Read the model definition and answer for the solid it produces. Units are mm, in the model's axes. A direction names the side the tool comes from. Coordinates: 2 decimals unless noted, no trailing zeros. Write each loop counter-clockwise with the first axis right and the second up, starting at its lowest first coordinate (ties: lowest second). Pieces come first, ordered by that corner, then holes.
Item 1: Section B-B (y = 7) is taken. Give the vertices of the cut face in (x, z), then the cut area to 3 significant figures.
Item 2: Each of these flat-tipped pins is pushed along its axis until it touches: P1, Ø3, axis at x = -1, y = 33, coming from the -Z side; P2, Ø1, axis at x = -4.5, y = 35, coming from the +Z side. Where does it stop, or does it pass through?
Item 3: A tool of negligible diameter and unlimited length cuts with its end or side. For faces 1 (the face through (7, 1, -43)), 2 (the face through (-6, 29, 40)), 3 (the face through (3.5, 2, 41)), 4 (the face through (3.5, 2, -41)), 5 (the face through (-6, 29, -40)), from which of +Z, -Z, +X, -X, +Y, -Y can it reach the whole face along a straight path? Write none if from no direction.
Item 4: Section A-A (x = 1.5) is taken. Give the vertices of the cut face in (y, z).
Item 5: Straight lines are drawn through the part: probe 1 along Z at (x, y) = (-2.5, 16); probe 2 along Y at (x, z) = (6, 39); probe 3 along X at (y, z) = (8, -39.5). For each, find the intervals that lie inside material, in ascending order.
from build123d import *

# Parameters (mm, degrees)
SKETCH1_W           = 20
SKETCH1_H           = 86
BOSS_EXTRUDE1_DEPTH = 3
CUT_EXTRUDE1_DEPTH  = 4
SKETCH3_W           = 4
SKETCH3_H           = 86
BOSS_EXTRUDE2_DEPTH = 52
SKETCH4_W           = 16
SKETCH4_H           = 74
BOSS_EXTRUDE3_DEPTH = 52


with BuildPart() as part:
    # Sketch1 → Boss-Extrude1 (new body)
    with BuildSketch(Plane(origin=(0, 0, 0), x_dir=(1, 0, 0), z_dir=(0, 1, 0))):
        Rectangle(SKETCH1_W, SKETCH1_H)
    extrude(amount=BOSS_EXTRUDE1_DEPTH)

    # Sketch2 → Cut-Extrude1 (cut, through all)
    with BuildSketch(Plane(origin=(0, 3, 0), x_dir=(1, 0, 0), z_dir=(0, 1, 0))):
        with BuildLine():
            Line((-0.5, 39.5), (-0.5, 43))
            Line((-0.5, 43), (3.5, 43))
            Line((3.5, 43), (3.5, 39.5))
            ThreePointArc((3.5, 39.5), (1.5, 37.5), (-0.5, 39.5))
        make_face()
        with BuildLine():
            Line((-0.5, -39.5), (-0.5, -43))
            Line((-0.5, -43), (3.5, -43))
            Line((3.5, -43), (3.5, -39.5))
            ThreePointArc((3.5, -39.5), (1.5, -37.5), (-0.5, -39.5))
        make_face()
    extrude(amount=-CUT_EXTRUDE1_DEPTH, mode=Mode.SUBTRACT)

    # Sketch3 → Boss-Extrude2 (add)
    with BuildSketch(Plane(origin=(0, 3, 0), x_dir=(1, 0, 0), z_dir=(0, 1, 0))):
        with Locations((-8, 0)):
            Rectangle(SKETCH3_W, SKETCH3_H)
    extrude(amount=BOSS_EXTRUDE2_DEPTH)

    # Sketch4 → Boss-Extrude3 (add)
    with BuildSketch(Plane(origin=(0, 3, 0), x_dir=(1, 0, 0), z_dir=(0, 1, 0))):
        with Locations((2, 0)):
            Rectangle(SKETCH4_W, SKETCH4_H)
    extrude(amount=BOSS_EXTRUDE3_DEPTH)


solid = part.part
Established:
1. outline: (-10, -43) - (-6, -43) - (-6, -37) - (10, -37) - (10, 37) - (-6, 37) - (-6, 43) - (-10, 43) - close
1. area: 1,530 mm2
2. P1: stops at z = -37
2. P2: stops at z = 37
3. face 1: -Z, +X, -X, +Y, -Y
3. face 2: +Z, +X, +Y
3. face 3: +Z, +Y, -Y
3. face 4: -Z, +Y, -Y
3. face 5: -Z, +X, +Y
4. outline: (0, -37.5) - (3, -37.5) - (3, -37) - (55, -37) - (55, 37) - (3, 37) - (3, 37.5) - (0, 37.5) - close
5. probe 1: z = -37 to 37
5. probe 2: y = 0 to 3
5. probe 3: x = -10 to -6
